Check sheet for the modelled part. Datum: model origin and axes. Units: mm. Face numbers are marked on the shaded views. A direction names the side the tool comes from. Round coordinates to 2 decimals unless told otherwise and drop trailing zeros. Write each loop counter-clockwise with the first axis right and the second up, starting at its lowest first coordinate (ties: lowest second). Pieces come first, ordered by that corner, then holes. Notation, with made-up numbers: (-19.75, -15) -> (3.25, -15) arc R20 ccw to (3.25, 9) -> close; hole circle Ø2 at (-28.75, -4.75). An arc over 180 degrees is marked (long way). Put each result on its own line as item: value. Start each with the question number.
from build123d import *

# Parameters (mm, degrees)
F0_R     = 2.032
F0_R_2   = 7.7573632
F1_DEPTH = 6.35
F3_R     = 10.2235
F3_R_2   = 7.7573632
F4_DEPTH = 6.35
F6_R     = 18.5400007717
F6_R_2   = 16
F7_DEPTH = 12.7
F13_R    = 5.08


with BuildPart() as f1:
    # F0 (on Top) → F1 (new body)
    with BuildSketch(Plane.XY):
        with BuildLine():
            Line((-41.275, -1.3013436), (-41.275, -29.21))
            ThreePointArc((-41.275, -29.21), (-40.5310512242, -31.0060512242), (-38.735, -31.75))
            Line((-38.735, -31.75), (38.735, -31.75))
            ThreePointArc((38.735, -31.75), (40.5310512242, -31.0060512242), (41.275, -29.21))
            Line((41.275, -29.21), (41.275, 29.21))
            ThreePointArc((41.275, 29.21), (40.5310512242, 31.0060512242), (38.735, 31.75))
            Line((38.735, 31.75), (-26.1691374, 31.75))
            ThreePointArc((-26.1691374, 31.75), (-27.9651886242, 31.0060512242), (-28.7091374, 29.21))
            Line((-28.7091374, 29.21), (-28.7091374, 3.7786564))
            ThreePointArc((-28.7091374, 3.7786564), (-29.4530861758, 1.9826051758), (-31.2491374, 1.2386564))
            Line((-31.2491374, 1.2386564), (-38.735, 1.2386564))
            ThreePointArc((-38.735, 1.2386564), (-40.5310512242, 0.4947076242), (-41.275, -1.3013436))
        make_face()
        with Locations((-34.925, -25.4)):
            Circle(F0_R, mode=Mode.SUBTRACT)
        with Locations((-9.525, -19.05)):
            Circle(F0_R, mode=Mode.SUBTRACT)
        with Locations((34.925, -25.4)):
            Circle(F0_R, mode=Mode.SUBTRACT)
        with Locations((-9.525, 6.35)):
            Circle(F0_R_2, mode=Mode.SUBTRACT)
        with Locations((34.925, 12.7)):
            Circle(F0_R, mode=Mode.SUBTRACT)
    extrude(amount=F1_DEPTH)

    # F3 (on face) → F4 (join)
    with BuildSketch(Plane.XY.offset(6.35)):
        with Locations((-9.525, 6.35)):
            Circle(F3_R)
        with Locations((-9.525, 6.35)):
            Circle(F3_R_2, mode=Mode.SUBTRACT)
    extrude(amount=F4_DEPTH)



with BuildPart() as f7:
    # F6 (on offset) → F7 (new body)
    with BuildSketch(Plane.XY.offset(31.75)):
        with Locations((-9.525, 6.35)):
            Circle(F6_R)
        with Locations((-9.525, 6.35)):
            Circle(F6_R_2, mode=Mode.SUBTRACT)
    extrude(amount=F7_DEPTH)


with BuildPart() as f1_1:
    add(f1.part)

    add(f7.part)  # F12 merges F7
    # F11 (on 3pt) → F12 (revolve)
    with BuildSketch(Plane.XZ.offset(-6.35)):
        with BuildLine():
            Line((9.0150007717, 31.75), (6.475, 31.75))
            Line((6.475, 31.75), (-1.5546870253, 13.7024863815))
            ThreePointArc((-1.5546870253, 13.7024863815), (-1.7138119778, 13.2124272026), (-1.7676368, 12.7))
            Line((-1.7676368, 12.7), (0.6985, 12.7))
            Line((0.6985, 12.7), (8.7917948258, 30.7088152634))
            ThreePointArc((8.7917948258, 30.7088152634), (8.9585724839, 31.2175794543), (9.0150007717, 31.75))
        make_face()
    revolve(axis=Axis((-9.525, 6.35, 28.575), (0, 0, -1)))

    # F13
    f13_edges = [f1_1.edges().sort_by_distance(p)[0] for p in [
        (-19.7485, 6.35, 12.7),
        (-19.7485, 6.35, 6.35),
        (-25.525, 6.35, 31.75),
    ]]
    fillet(f13_edges, radius=F13_R)


solid = f1_1.part
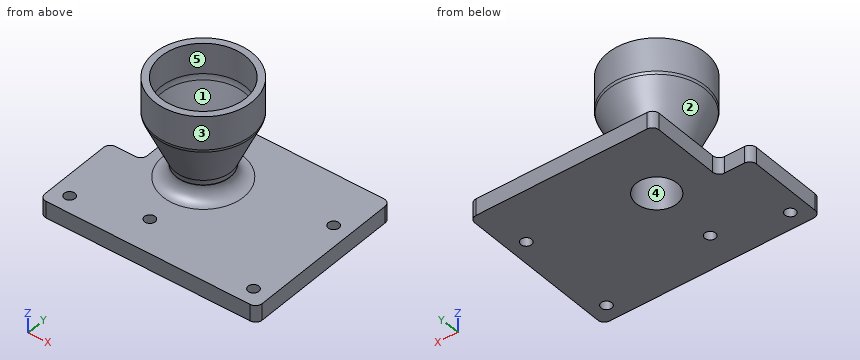
1. Material ranges on L1, parallel to X at y = 6, z = 37; L2, parallel to Z at x = 24, y = 0; L3, parallel to X at y = -2, z = 41.5, recorded low to high. Write a range as [from, to].
2. Section check B-B, the plane z = 37.5. Enter the section's corners in (x, y) (3 decimals).
3. Draft check along Z on the marked faces 1, 2 and 3. Enter one of: released by +Z, released by -Z, zero draft, split by the parting line, or undercut.
4. Section check A-A, the plane y = -25.4. Enter the section's corners in (x, z) (3 decimals), then the cut area to 3 significant figures.
5. Gauge pin test, flat ends, axial feed: P1, Ø12, axis at x = -21, z = 21.5, coming from the -Y side; P2, Ø3, axis at y = 1, z = 18.5, coming from the -X side; P3, Ø4.5, axis at x = 34.925, y = -25.4, coming from the +Z side; P4, Ø3.5, axis at x = -9.525, y = -19.05, coming from the +Z side (3 decimals). Record the tip position at first contact, or that the pin passes through.
6. Section check D-D, the plane y = -15.5. Enter the section's corners in (x, z) (3 decimals).
7. Access from +Z, -Z, +X, -X, +Y, -Y to the whole of each face (thin tool, end or side, straight path). Record for the marked faces 4 and 5.
8. Section check C-C, the plane x = 31. Enter the section's corners in (y, z).
Reply:
1. L1: x = [-28.06, -25.52], [6.47, 9.01]
1. L2: z = [0, 6.35]
1. L3: x = [-26.08, -23.17], [4.12, 7.03]
2. outline: circle Ø37.08 at (-9.525, 6.35); hole circle Ø32 at (-9.525, 6.35)
3. face 1: released by +Z
3. face 2: undercut
3. face 3: zero draft
4. outline: (-41.275, 0) -> (-36.957, 0) -> (-36.957, 6.35) -> (-41.275, 6.35) -> close; (-32.893, 0) -> (32.893, 0) -> (32.893, 6.35) -> (-32.893, 6.35) -> close; (36.957, 0) -> (41.275, 0) -> (41.275, 6.35) -> (36.957, 6.35) -> close
4. area: 473 mm2
5. P1: stops at y = -8.02
5. P2: stops at x = -22.13
5. P3: stops at z = 6.35
5. P4: passes through
6. outline: (-41.275, 0) -> (41.275, 0) -> (41.275, 6.35) -> (-41.275, 6.35) -> close
7. face 4: +Z, -Z
7. face 5: +Z
8. outline: (-31.75, 0) -> (31.75, 0) -> (31.75, 6.35) -> (-31.75, 6.35) -> close
